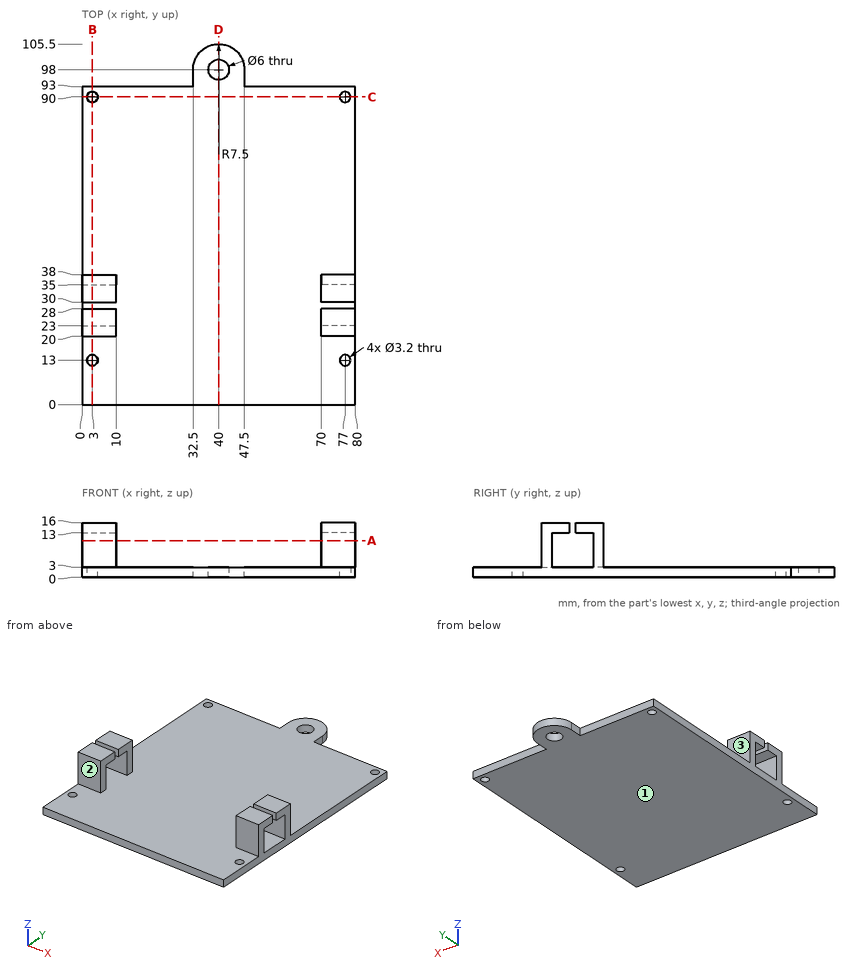
Study the drawing (mm; zero at the part's minimum x, y, z) and answer. A direction names the side the tool comes from. Give positions to 0.01 mm unless a question says otherwise; leave off trailing zeros. Order: outer loops, then holes, each group sorted by start corner. A loop starts at its lowest first (then second) coordinate and runs counter-clockwise, first axis right, second up. Notation, with made-up numbers: (42.25, 3) - (48.25, 3) arc R12 ccw to (48.25, 12) - close; hole circle Ø3 at (-26, 23.25). An arc over 180 degrees is marked (long way). Answer in a Markdown table with one row per item. Add a question column.
Q1. The part is cut by section D-D (x = 40). Determine the outline of the cut face in (y, z), then the cut area to 4 significant figures.
Q2. The part is cut by section C-C (y = 90). Determine the outline of the cut face in (x, z).
Q3. The part is cut by section B-B (x = 3). Determine the outline of the cut face in (y, z).
Q4. Find the intervals of material crossed by line 1 along Y through (x, z) = (3, 2); line 2 along X through (y, z) = (90, 0.75); line 3 along Y through (x, z) = (40, 0.95), in increasing order. Write a range as [from, to].
Q5. Which of the six approach directions +Z, -Z, +X, -X, +Y, -Y give full straight-line access (tool end or side, diameter ignored) to the marked faces 1, 2 and 3?
Q6. Given P1, Ø5, axis at x = 4.5, z = 9, coming from the +Y side; P2, Ø1.9, axis at x = 3, y = 90, coming from the +Z side; P3, Ø3.5, axis at x = 16.5, z = 2, coming from the +Y side; P4, Ø6, axis at x = 30, y = 88.5, coming from the +Z side, each flat-ended and moving along its own axis, determine where each tip first touches the part or whether it passes through.
Q7. The part is cut by section A-A (z = 10.75). Determine the outline of the cut face in (x, y), then the cut area to 3 significant figures.
Determined:
| question | item | result |
|---|---|---|
| 1 | outline | (0, 0) - (95, 0) - (95, 3) - (0, 3) - close; (101, 0) - (105.5, 0) - (105.5, 3) - (101, 3) - close |
| 1 | area | 298.5 mm² |
| 2 | outline | (0, 0) - (1.4, 0) - (1.4, 3) - (0, 3) - close; (4.6, 0) - (75.4, 0) - (75.4, 3) - (4.6, 3) - close; (78.6, 0) - (80, 0) - (80, 3) - (78.6, 3) - close |
| 3 | outline | (0, 0) - (11.4, 0) - (11.4, 3) - (0, 3) - close; (14.6, 0) - (88.4, 0) - (88.4, 3) - (38, 3) - (38, 16) - (30, 16) - (30, 13) - (35, 13) - (35, 3) - (23, 3) - (23, 13) - (28, 13) - (28, 16) - (20, 16) - (20, 3) - (14.6, 3) - close; (91.6, 0) - (93, 0) - (93, 3) - (91.6, 3) - close |
| 4 | line 1 | y = [0, 11.4], [14.6, 88.4], [91.6, 93] |
| 4 | line 2 | x = [0, 1.4], [4.6, 75.4], [78.6, 80] |
| 4 | line 3 | y = [0, 95], [101, 105.5] |
| 5 | face 1 | -Z, +X, -X, +Y, -Y |
| 5 | face 2 | +Z, +X, -X, -Y |
| 5 | face 3 | +Z, +X, -X, +Y |
| 6 | P1 | stops at y = 38 |
| 6 | P2 | passes through |
| 6 | P3 | stops at y = 93 |
| 6 | P4 | stops at z = 3 |
| 7 | outline | (0, 20) - (10, 20) - (10, 23) - (0, 23) - close; (0, 35) - (10, 35) - (10, 38) - (0, 38) - close; (70, 20) - (80, 20) - (80, 23) - (70, 23) - close; (70, 35) - (80, 35) - (80, 38) - (70, 38) - close |
| 7 | area | 120 mm² |
